Autodesk Fusion 360 part; units mm, degrees
sketch "Sketch1" plane through (0, 0, 0) normal (0, 0, 1) x (1, 0, 0) in component "fidget spinner"
  circle A0 centre (0, 0) radius 4
  circle A1 centre (0, 0) radius 11
  circle A2 centre (0, 0) radius 13.5
  line L0 (-3.7528, 42.5) -> (-7.5056, 36)
  line L1 (-7.5056, 36) -> (-3.7528, 29.5)
  line L2 (-3.7528, 29.5) -> (3.7528, 29.5)
  line L3 (3.7528, 29.5) -> (7.5056, 36)
  line L4 (7.5056, 36) -> (3.7528, 42.5)
  line L5 (3.7528, 42.5) -> (-3.7528, 42.5)
  line L6 (-12.6841, 7.3232) -> (-8.9294, 37.125)
  line L7 (12.6841, 7.3232) -> (8.9294, 37.125)
  line L8 (-34.9297, -11.5) -> (-38.6825, -18)
  line L9 (-38.6825, -18) -> (-34.9297, -24.5)
  line L10 (-34.9297, -24.5) -> (-27.4241, -24.5)
  line L11 (-27.4241, -24.5) -> (-23.6714, -18)
  line L12 (-23.6714, -18) -> (-27.4241, -11.5)
  line L13 (-27.4241, -11.5) -> (-34.9297, -11.5)
  line L14 (0, -14.6463) -> (-27.6865, -26.2956)
  line L15 (-12.6841, 7.3232) -> (-36.6159, -10.8294)
  line L16 (27.4241, -24.5) -> (34.9297, -24.5)
  line L17 (34.9297, -24.5) -> (38.6825, -18)
  line L18 (38.6825, -18) -> (34.9297, -11.5)
  line L19 (34.9297, -11.5) -> (27.4241, -11.5)
  line L20 (27.4241, -11.5) -> (23.6714, -18)
  line L21 (23.6714, -18) -> (27.4241, -24.5)
  line L22 (12.6841, 7.3232) -> (36.6159, -10.8294)
  line L23 (0, -14.6463) -> (27.6865, -26.2956)
  arc A3 (8.9294, 37.125) -> (-8.9294, 37.125) centre (0, 36) ccw
  arc A4 (-36.6159, -10.8294) -> (-27.6865, -26.2956) centre (-31.1769, -18) ccw
  arc A5 (27.6865, -26.2956) -> (36.6159, -10.8294) centre (31.1769, -18) ccw
  point P0 (0, 36)
  dimension "d1" = 8
  dimension "d2" = 22
  dimension "d3" = 27
  dimension "d4" = 36
  dimension "d5" = 6.5
  dimension "d6" = 18
extrude "Extrude1" add sketch "Sketch1" along normal mid plane 8 contours A2 | L6 L7 L14 L15 L22 L23 A3 A4 A5 in component "fidget spinner"
component "fidget spinner" placed x (1, 0, 0) y (0, 1, 0) z (0, 0, 1) at (0, 0, 0)
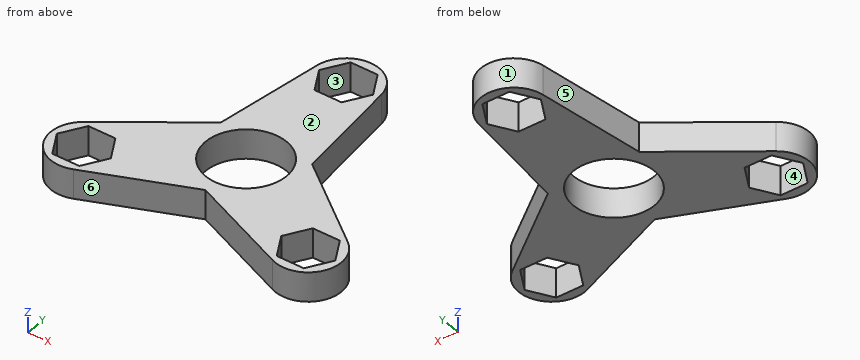
Check sheet for the modelled part. Datum: model origin and axes. Units: mm. Face numbers are marked on the shaded views. A direction names the side the tool comes from. Give positions to 0.01 mm unless a question says otherwise; leave off trailing zeros. Write each loop counter-clockwise with the first axis right and the second up, starting at its lowest first coordinate (ties: lowest second). Pieces come first, ordered by that corner, then holes. Notation, with made-up numbers: (-38, 13.25) - (9, 13.25) arc R4 ccw to (9, 19.25) - close; hole circle Ø6 at (-24, 59). An arc over 180 degrees is marked (long way). Answer as a JSON object with one key per item and string values. Group by question number.
1) Thickness scan on probe 1 along Y at (x, z) = (0, 1.75); probe 2 along X at (y, z) = (-16, -1.5); probe 3 along X at (y, z) = (-20, 1.75). Record the ranges inside material, lowest first. Write a range as from..to.
2) Release check for a two-part mould opening along X. For the marked faces 1, 2 and 3 record: pulls with the +X half, pulls with the -X half, needs draft (parallel to the pull), parting line crosses it, or undercut.
3) Sectioned sample at D-D (x = 25.5). Record the cut outline in (y, z), then the cut area to 3 significant figures.
4) Sectioned sample at A-A (x = -1). Record the cut outline in (y, z), then the cut area to 3 significant figures.
5) Sectioned sample at C-C (y = -13.5). Record the cut outline in (x, z), then the cut area to 3 significant figures.
6) Sectioned sample at B-B (z = 0.25). Record the cut outline in (x, y) (1 decimal), then the cut area to 3 significant figures.
7) Depth check by flat-ended pin: P1, Ø4, axis at x = -23.5, z = 0, coming from the +Y side; P2, Ø1.5, axis at x = -17, z = -0.5, coming from the +Y side; P3, Ø2, axis at y = -2.5, z = 1.5, coming from the +X side. Enter the tip coordinate at first touch or a pass-through.
8) Access from +Z, -Z, +X, -X, +Y, -Y to the whole of each face (thin tool, end or side, straight path). Record for the marked faces 4, 5 and 6.
Geometry results:
{
 "1": {"probe 1": "y = -14.65..-11, 11..29.5, 42.5..45", "probe 2": "x = -39.95..-37.53, -24.83..-3.22, 3.22..24.83, 37.53..39.95", "probe 3": "x = -39.95..-37.53, -24.83..-12.72, 12.72..24.83, 37.53..39.95"},
 "2": {"face 1": "parting line crosses it", "face 2": "needs draft", "face 3": "undercut"},
 "3": {"outline": "(-25.38, -4) - (-21.17, -4) - (-21.17, 4) - (-25.38, 4) - close; (-14.83, -4) - (-2.4, -4) - (-2.4, 4) - (-14.83, 4) - close", "area": "133 mm^2"},
 "4": {"outline": "(-15.07, -4) - (-10.95, -4) - (-10.95, 4) - (-15.07, 4) - close; (10.95, -4) - (29.5, -4) - (29.5, 4) - (10.95, 4) - close; (42.5, -4) - (44.94, -4) - (44.94, 4) - (42.5, 4) - close", "area": "201 mm^2"},
 "5": {"outline": "(-38.97, -4) - (-36.08, -4) - (-36.08, 4) - (-38.97, 4) - close; (-26.27, -4) - (26.27, -4) - (26.27, 4) - (-26.27, 4) - close; (36.08, -4) - (38.97, -4) - (38.97, 4) - (36.08, 4) - close", "area": "466 mm^2"},
 "6": {"outline": "(-36.6, -10.8) arc R9 ccw to (-27.7, -26.3) - (0, -14.6) - (27.7, -26.3) arc R9 ccw to (36.6, -10.8) - (12.7, 7.3) - (8.9, 37.1) arc R9 ccw to (-8.9, 37.1) - (-12.7, 7.3) - close; hole (-38.7, -18) - (-34.9, -24.5) - (-27.4, -24.5) - (-23.7, -18) - (-27.4, -11.5) - (-34.9, -11.5) - close; hole circle Ø22 at (0, 0); hole (-7.5, 36) - (-3.8, 29.5) - (3.8, 29.5) - (7.5, 36) - (3.8, 42.5) - (-3.8, 42.5) - close; hole (23.7, -18) - (27.4, -24.5) - (34.9, -24.5) - (38.7, -18) - (34.9, -11.5) - (27.4, -11.5) - close", "area": "1,710 mm^2"},
 "7": {"P1": "stops at y = 0.64", "P2": "stops at y = 4.62", "P3": "stops at x = 26.95"},
 "8": {"face 4": "+Z, -Z", "face 5": "+Z, -Z, -X, +Y", "face 6": "+Z, -Z, -Y"}
}
